Can you work these out from the drawing? Everything is in mm from the part's minimum corner. A direction names the side the tool comes from. Coordinates: 2 decimals unless noted, no trailing zeros. Order: outer loops, then holes, each group sorted by start corner. A loop starts at its lowest first (then second) coordinate and runs counter-clockwise, first axis right, second up. Notation, with made-up numbers: (72.5, -7.5) - (80.5, -7.5) arc R9 ccw to (80.5, -2.5) - close; hole circle Ø9 at (20, 82.5). An arc over 180 degrees is marked (long way). Use a Markdown table: item, result. Add a question column.
(1) I want a section at A-A (x = 5). List the corners of the cut face in (y, z) for me, and give its area (3 significant figures).
(2) For pin 1 Ø3 at (x, y) = (59, 14) entering from +Z; pin 2 Ø4 at (y, z) = (2.5, 8) entering from -X; pin 3 Ø3 at (x, y) = (5, 20) entering from -Z; pin 4 Ø4 at (y, z) = (14, 12) entering from +X, each with a flat end and sliding along its axis, tell me the tip position at first contact or that it passes through.
(3) On a 3-axis mill with a long thin cutter (end or side, diameter ignored), from which of +Z, -Z, +X, -X, +Y, -Y can I reach the whole of each face in a straight line? I mean the marked faces 4, 5 and 6. Say none if no direction works.
(4) I want a section at D-D (y = 2.25). List the corners of the cut face in (x, z) for me.
(5) If I drill on L1, parallel to Y at x = 5, z = 1.95; L2, parallel to X at y = 11.5, z = 10.75; L3, parallel to Z at x = 60, y = 14.5, over which ranges is the centre line in solid material (lowest first)? Write a range as [from, to].
(6) I want a section at C-C (z = 7.75). List the corners of the cut face in (x, y) for me.
(7) We'd pull the mould along X, two halves only. Please class the marked faces 1, 2 and 3: pulls with the +X half, pulls with the -X half, needs draft (parallel to the pull), parting line crosses it, or undercut.
(8) I want a section at B-B (y = 5). List the corners of the cut face in (x, z) for me, and give its area (3 significant figures).
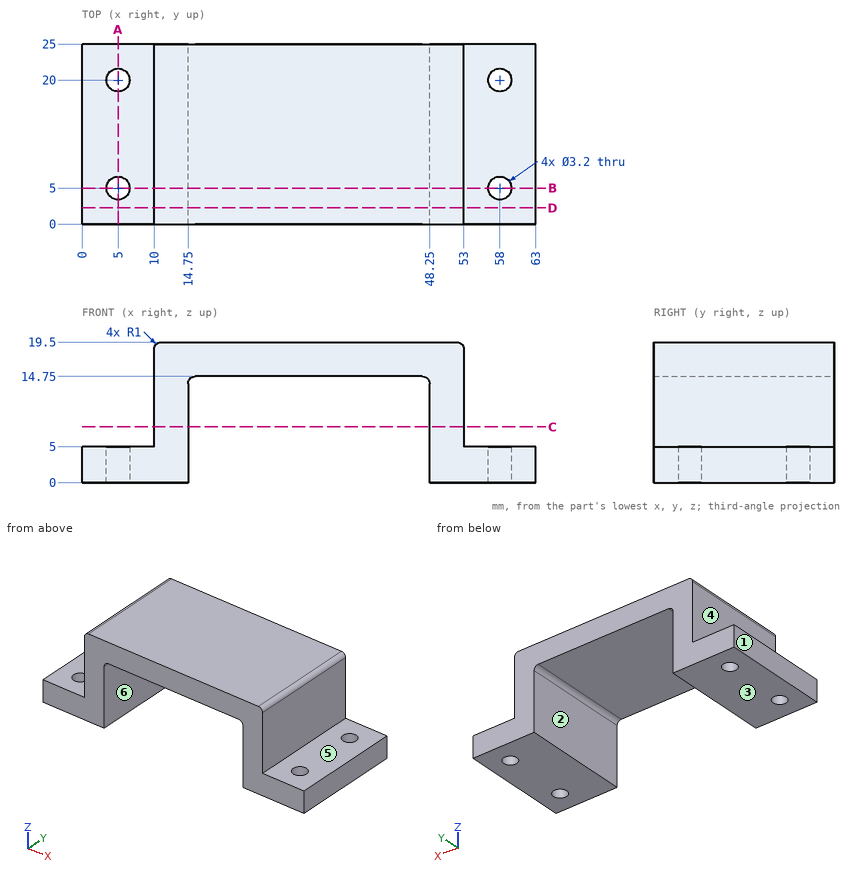
Answers follow:
| question | item | result |
|---|---|---|
| 1 | outline | (0, 0) - (3.4, 0) - (3.4, 5) - (0, 5) - close; (6.6, 0) - (18.4, 0) - (18.4, 5) - (6.6, 5) - close; (21.6, 0) - (25, 0) - (25, 5) - (21.6, 5) - close |
| 1 | area | 93.0 mm² |
| 2 | pin 1 | stops at z = 5 |
| 2 | pin 2 | stops at x = 10 |
| 2 | pin 3 | passes through |
| 2 | pin 4 | stops at x = 53 |
| 3 | face 4 | +Z, -X, +Y, -Y |
| 3 | face 5 | +Z, +X, +Y, -Y |
| 3 | face 6 | -Z, +Y, -Y |
| 4 | outline | (0, 0) - (14.75, 0) - (14.75, 13.75) arc R1 cw to (15.75, 14.75) - (47.25, 14.75) arc R1 cw to (48.25, 13.75) - (48.25, 0) - (63, 0) - (63, 5) - (53, 5) - (53, 18.5) arc R1 ccw to (52, 19.5) - (11, 19.5) arc R1 ccw to (10, 18.5) - (10, 5) - (0, 5) - close |
| 5 | L1 | y = [0, 3.4], [6.6, 18.4], [21.6, 25] |
| 5 | L2 | x = [10, 14.75], [48.25, 53] |
| 5 | L3 | z = [0, 5] |
| 6 | outline | (10, 0) - (14.75, 0) - (14.75, 25) - (10, 25) - close; (48.25, 0) - (53, 0) - (53, 25) - (48.25, 25) - close |
| 7 | face 1 | pulls with the -X half |
| 7 | face 2 | undercut |
| 7 | face 3 | needs draft |
| 8 | outline | (0, 0) - (3.4, 0) - (3.4, 5) - (0, 5) - close; (6.6, 0) - (14.75, 0) - (14.75, 13.75) arc R1 cw to (15.75, 14.75) - (47.25, 14.75) arc R1 cw to (48.25, 13.75) - (48.25, 0) - (56.4, 0) - (56.4, 5) - (53, 5) - (53, 18.5) arc R1 ccw to (52, 19.5) - (11, 19.5) arc R1 ccw to (10, 18.5) - (10, 5) - (6.6, 5) - close; (59.6, 0) - (63, 0) - (63, 5) - (59.6, 5) - close |
| 8 | area | 412 mm² |
